```python
from build123d import *

# Parameters (mm, degrees)
BOSS_EXTRUDE1_DEPTH        = 1.6
F_3_2_3_2_DIAMETER_HOLE1_D = 3.2
FILLET1_R                  = 3
FILLET2_R                  = 1
FILLET3_R                  = 2


with BuildPart() as part:
    # Sketch1 → Boss-Extrude1 (new body)
    with BuildSketch(Plane.XY):
        Polygon((-72.5, 0.75), (-72.5, 5.75), (-6.5, 5.75), (-6.5, 0.75), (6.5, 0.75), (6.5, 92.75), (-85.5, 92.75), (-85.5, 54.75), (-81.5, 54.75), (-81.5, 38.75), (-85.5, 38.75), (-85.5, 0.75), align=None)
    extrude(amount=-BOSS_EXTRUDE1_DEPTH)

    # Ø3.2 (3.2) Diameter Hole1 (through all)
    with Locations(Plane(origin=(0, 0, -1.6), x_dir=(-1, 0, 0), z_dir=(0, 0, -1))):
        with Locations((1.5, 84.75), (1.5, 8.75), (77.5, 8.75), (77.5, 84.75)):
            Hole(F_3_2_3_2_DIAMETER_HOLE1_D / 2)

    # Fillet1
    fillet1_edges = [part.edges().sort_by_distance(p)[0] for p in [
        (6.5, 0.75, -0.8),
        (-6.5, 5.75, -0.8),
        (-72.5, 5.75, -0.8),
        (-85.5, 0.75, -0.8),
        (-85.5, 92.75, -0.8),
        (6.5, 92.75, -0.8),
    ]]
    fillet(fillet1_edges, radius=FILLET1_R)

    # Fillet2
    fillet2_edges = [part.edges().sort_by_distance(p)[0] for p in [
        (-6.5, 0.75, -0.8),
        (-72.5, 0.75, -0.8),
        (-85.5, 38.75, -0.8),
        (-85.5, 54.75, -0.8),
    ]]
    fillet(fillet2_edges, radius=FILLET2_R)

    # Fillet3
    fillet3_edges = [part.edges().sort_by_distance(p)[0] for p in [
        (-81.5, 38.75, -0.8),
        (-81.5, 54.75, -0.8),
    ]]
    fillet(fillet3_edges, radius=FILLET3_R)


solid = part.part
```
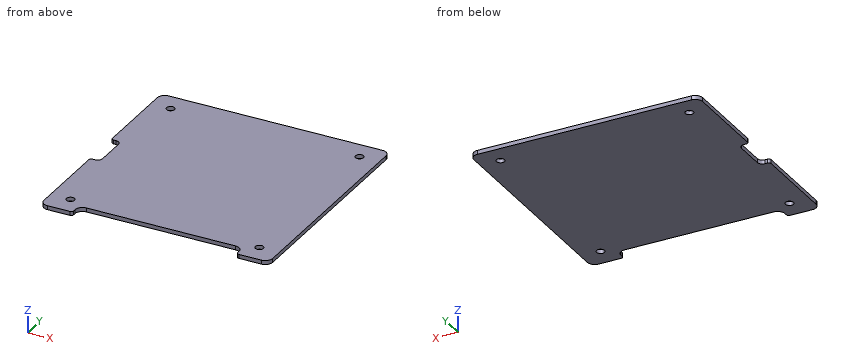
The model under review builds one solid part; all positions refer to its coordinate system, in mm. Give positions to 0.01 mm unless a question says otherwise; leave off trailing zeros. Loops run counter-clockwise (first coordinate to the right, second up) from the corner with the lowest first, then second, coordinate; pieces in that order, holes last. Notation, with made-up numbers: (47.25, 74.5) - (93.25, 74.5) arc R13 ccw to (93.25, 94.5) - close; hole circle Ø11 at (36.25, 81). An arc over 180 degrees is marked (long way). Answer as a JSON object with one key per item and string values.
Q1. To check wall thickness, follow line 1 along Y through (x, z) = (-1.5, -1.2); line 2 along X through (y, z) = (84.75, -1.2); line 3 along Y through (x, z) = (-47, -0.9). State the ranges of each line that lie inside material, in increasing order.
Worked out:
{"line 1": "y = 0.75 to 7.15, 10.35 to 83.15, 86.35 to 92.75", "line 2": "x = -85.5 to -79.1, -75.9 to -3.1, 0.1 to 6.5", "line 3": "y = 5.75 to 92.75"}
Q2. Insertion check: pin 1 (0.5 mm diameter, centred on y = 2.5, z = -1, fed in from +X); pin 2 (0.8 mm diameter, centred on y = 46.5, z = -1, fed in from -X); pin 3 (0.8 mm diameter, centred on x = -84, z = -0.5, fed in from +Y). Each pin has a flat end and moves straight along its axis. Give the tip position at first contact, or say it passes through.
Worked out:
{"pin 1": "stops at x = 6.33", "pin 2": "stops at x = -81.5", "pin 3": "stops at y = 92.54"}
Q3. Add section B-B on y = 84.75. State the section outline as (x, z) points.
Worked out:
{"outline": "(-85.5, -1.6) - (-79.1, -1.6) - (-79.1, 0) - (-85.5, 0) - close; (-75.9, -1.6) - (-3.1, -1.6) - (-3.1, 0) - (-75.9, 0) - close; (0.1, -1.6) - (6.5, -1.6) - (6.5, 0) - (0.1, 0) - close"}
Q4. Add section C-C on z = -0.8. State the section outline as (x, y) points.
Worked out:
{"outline": "(-85.5, 3.75) arc R3 ccw to (-82.5, 0.75) - (-73.5, 0.75) arc R1 ccw to (-72.5, 1.75) - (-72.5, 2.75) arc R3 cw to (-69.5, 5.75) - (-9.5, 5.75) arc R3 cw to (-6.5, 2.75) - (-6.5, 1.75) arc R1 ccw to (-5.5, 0.75) - (3.5, 0.75) arc R3 ccw to (6.5, 3.75) - (6.5, 89.75) arc R3 ccw to (3.5, 92.75) - (-82.5, 92.75) arc R3 ccw to (-85.5, 89.75) - (-85.5, 55.75) arc R1 ccw to (-84.5, 54.75) - (-83.5, 54.75) arc R2 cw to (-81.5, 52.75) - (-81.5, 40.75) arc R2 cw to (-83.5, 38.75) - (-84.5, 38.75) arc R1 ccw to (-85.5, 37.75) - close; hole circle Ø3.2 at (-77.5, 8.75); hole circle Ø3.2 at (-77.5, 84.75); hole circle Ø3.2 at (-1.5, 8.75); hole circle Ø3.2 at (-1.5, 84.75)"}
Q5. Add section A-A on x = -77.5. State the section outline as (y, z) points.
Worked out:
{"outline": "(0.75, -1.6) - (7.15, -1.6) - (7.15, 0) - (0.75, 0) - close; (10.35, -1.6) - (83.15, -1.6) - (83.15, 0) - (10.35, 0) - close; (86.35, -1.6) - (92.75, -1.6) - (92.75, 0) - (86.35, 0) - close"}
Q6. Add section D-D on x = -23. State the section outline as (y, z) points, plus the area to 3 significant figures.
Worked out:
{"outline": "(5.75, -1.6) - (92.75, -1.6) - (92.75, 0) - (5.75, 0) - close", "area": "139 mm^2"}
